from build123d import *

# Parameters (mm, degrees)
BOSS_EXTRUDE1_DEPTH = 4
SKETCH3_W           = 286.6
SKETCH3_H           = 12
BOSS_EXTRUDE2_DEPTH = 4
CUT_EXTRUDE1_REACH  = 258.811
SKETCH4_R           = 1.55


with BuildPart() as part:
    # Sketch1 → Boss-Extrude1 (new body)
    with BuildSketch(Plane.XY):
        with BuildLine():
            Line((-4.65, 0), (-4.65, 4.65))
            Line((-4.65, 4.65), (-30.85, 4.65))
            Line((-30.85, 4.65), (-30.85, -15.35))
            Line((-30.85, -15.35), (255.75, -15.35))
            Line((255.75, -15.35), (255.75, 4.65))
            Line((255.75, 4.65), (243.35, 4.65))
            Line((243.35, 4.65), (243.35, 0))
            ThreePointArc((243.35, 0), (238.7, -4.65), (234.05, 0))
            Line((234.05, 0), (234.05, 4.65))
            Line((234.05, 4.65), (221.65, 4.65))
            Line((221.65, 4.65), (221.65, 0))
            ThreePointArc((221.65, 0), (217, -4.65), (212.35, 0))
            Line((212.35, 0), (212.35, 4.65))
            Line((212.35, 4.65), (199.95, 4.65))
            Line((199.95, 4.65), (199.95, 0))
            ThreePointArc((199.95, 0), (195.3, -4.65), (190.65, 0))
            Line((190.65, 0), (190.65, 4.65))
            Line((190.65, 4.65), (178.25, 4.65))
            Line((178.25, 4.65), (178.25, 0))
            ThreePointArc((178.25, 0), (173.6, -4.65), (168.95, 0))
            Line((168.95, 0), (168.95, 4.65))
            Line((168.95, 4.65), (156.55, 4.65))
            Line((156.55, 4.65), (156.55, 0))
            ThreePointArc((156.55, 0), (151.9, -4.65), (147.25, 0))
            Line((147.25, 0), (147.25, 4.65))
            Line((147.25, 4.65), (134.85, 4.65))
            Line((134.85, 4.65), (134.85, 0))
            ThreePointArc((134.85, 0), (130.2, -4.65), (125.55, 0))
            Line((125.55, 0), (125.55, 4.65))
            Line((125.55, 4.65), (113.15, 4.65))
            Line((113.15, 4.65), (113.15, 0))
            ThreePointArc((113.15, 0), (108.5, -4.65), (103.85, 0))
            Line((103.85, 0), (103.85, 4.65))
            Line((103.85, 4.65), (91.45, 4.65))
            Line((91.45, 4.65), (91.45, 0))
            ThreePointArc((91.45, 0), (86.8, -4.65), (82.15, 0))
            Line((82.15, 0), (82.15, 4.65))
            Line((82.15, 4.65), (69.75, 4.65))
            Line((69.75, 4.65), (69.75, 0))
            ThreePointArc((69.75, 0), (65.1, -4.65), (60.45, 0))
            Line((60.45, 0), (60.45, 4.65))
            Line((60.45, 4.65), (48.05, 4.65))
            Line((48.05, 4.65), (48.05, 0))
            ThreePointArc((48.05, 0), (43.4, -4.65), (38.75, 0))
            Line((38.75, 0), (38.75, 4.65))
            Line((38.75, 4.65), (26.35, 4.65))
            Line((26.35, 4.65), (26.35, 0))
            ThreePointArc((26.35, 0), (21.7, -4.65), (17.05, 0))
            Line((17.05, 0), (17.05, 4.65))
            Line((17.05, 4.65), (4.65, 4.65))
            Line((4.65, 4.65), (4.65, 0))
            ThreePointArc((4.65, 0), (0, -4.65), (-4.65, 0))
        make_face()
    extrude(amount=BOSS_EXTRUDE1_DEPTH)

    # Sketch3 → Boss-Extrude2 (add)
    with BuildSketch(Plane.XZ.offset(15.35)):
        with Locations((112.45, -6)):
            Rectangle(SKETCH3_W, SKETCH3_H)
    extrude(amount=-BOSS_EXTRUDE2_DEPTH)

    # Sketch4 → Cut-Extrude1 (cut, up to next)
    with BuildSketch(Plane.XZ.offset(15.35), mode=Mode.PRIVATE) as cut_extrude1_sk1:
        with Locations((-23.35, -4)):
            Circle(SKETCH4_R)
    cut_extrude1_tool1 = extrude(cut_extrude1_sk1.sketch, amount=-CUT_EXTRUDE1_REACH, mode=Mode.PRIVATE) & part.part
    # Sketch4 → Cut-Extrude1 (cut, up to next)
    with BuildSketch(Plane.XZ.offset(15.35), mode=Mode.PRIVATE) as cut_extrude1_sk2:
        with Locations((248.25, -4)):
            Circle(SKETCH4_R)
    cut_extrude1_tool2 = extrude(cut_extrude1_sk2.sketch, amount=-CUT_EXTRUDE1_REACH, mode=Mode.PRIVATE) & part.part
    # Sketch4 → Cut-Extrude1 (cut, up to next)
    with BuildSketch(Plane.XZ.offset(15.35), mode=Mode.PRIVATE) as cut_extrude1_sk3:
        with Locations((-9.85, -4)):
            Circle(SKETCH4_R)
    cut_extrude1_tool3 = extrude(cut_extrude1_sk3.sketch, amount=-CUT_EXTRUDE1_REACH, mode=Mode.PRIVATE) & part.part
    add(cut_extrude1_tool1.solids().sort_by_distance((-23.35, -15.35, -4))[0], mode=Mode.SUBTRACT)
    add(cut_extrude1_tool2.solids().sort_by_distance((248.25, -15.35, -4))[0], mode=Mode.SUBTRACT)
    add(cut_extrude1_tool3.solids().sort_by_distance((-9.85, -15.35, -4))[0], mode=Mode.SUBTRACT)


solid = part.part
Here's how the part is built. I have some questions about the finished solid (model axes, mm). A direction names the side the tool comes from. Coordinates: 2 decimals unless noted, no trailing zeros. Loops run counter-clockwise (first coordinate to the right, second up) from the corner with the lowest first, then second, coordinate; pieces in that order, holes last. Notation, with made-up numbers: (-15.5, 60.5) -> (14.5, 60.5) arc R25 ccw to (14.5, 95.5) -> close; hole circle Ø8 at (-20.5, -27). An arc over 180 degrees is marked (long way). Use one line per item in the form item = value. Start each with the question number.
(1) On a 3-axis mill with a long thin cutter (end or side, diameter ignored), from which of +Z, -Z, +X, -X, +Y, -Y can I reach the whole of each face in a straight line? I mean faces 1 (the face through (110, -11.35, -6)), 2 (the face through (65.2, -4.65, 1.97)). Say none if no direction works.
(2) If we section it at A-A (x = 86.8): Please give me the cut outline in (y, z), then the cut area to 3 significant figures.
(3) We'd pull the mould along X, two halves only. Please class faces 3 (the face through (110, -5, 0)), 4 (the face through (173.7, -4.65, 1.97)), 5 (the face through (-30.85, -10, 1)): pulls with the +X half, pulls with the -X half, needs draft (parallel to the pull), parting line crosses it, or undercut.
(4) Please list where these lines run through material, in increasing order: line 1 along Z through (x, y) = (-9.85, -13.25); line 2 along Z through (x, y) = (-5.5, -10.25); line 3 along Y through (x, z) = (128.5, -1).
(5) Will these pins go through, and if not, where does the flat tip stop? pin 1 (3 mm diameter, centred on x = 205.5, y = -8.5, fed in from -Z); pin 2 (5 mm diameter, centred on x = 220.5, y = -1.5, fed in from +Z); pin 3 (3 mm diameter, centred on x = 66.5, z = -10, fed in from +Y); pin 4 (3 mm diameter, centred on x = -23.35, z = -4, fed in from +Y).
Verdict:
q1.face_1 = -Z, +X, -X, +Y
q1.face_2 = +Z, -Z, +Y
q2.outline = (-15.35, -12) -> (-11.35, -12) -> (-11.35, 0) -> (-4.65, 0) -> (-4.65, 4) -> (-15.35, 4) -> close
q2.area = 90.8 mm²
q3.face_3 = needs draft
q3.face_4 = undercut
q3.face_5 = pulls with the -X half
q4.line_1 = -12 to -5.55, -2.45 to 4
q4.line_2 = 0 to 4
q4.line_3 = -15.35 to -11.35
q5.pin_1 = 0
q5.pin_2 = 4
q5.pin_3 = -11.35
q5.pin_4 = through
